from build123d import *

# Parameters (mm, degrees)
SKETCH1_W           = 26
SKETCH1_H           = 26
SKETCH1_R           = 1.5
BOSS_EXTRUDE1_DEPTH = 20
SKETCH2_R           = 10
SKETCH2_R_2         = 3
CUT_EXTRUDE1_DEPTH  = 15
SKETCH2_7_R         = 3
SKETCH2_7_R_2       = 1.5
CUT_EXTRUDE3_DEPTH  = 17
CHAMFER1_SIZE       = 1
BOSS_EXTRUDE3_DEPTH = 3.5


with BuildPart() as part:
    # Sketch1 → Boss-Extrude1 (new body)
    with BuildSketch(Plane.XY):
        with Locations((2.653979239, -3.148788927)):
            Rectangle(SKETCH1_W, SKETCH1_H)
        with Locations((2.653979239, 2.851211073)):
            Circle(SKETCH1_R, mode=Mode.SUBTRACT)
        with Locations((2.653979239, -9.148788927)):
            Circle(SKETCH1_R, mode=Mode.SUBTRACT)
    extrude(amount=BOSS_EXTRUDE1_DEPTH)

    # Sketch2 → Cut-Extrude1 (cut)
    with BuildSketch(Plane(origin=(0, 0, 0), x_dir=(-1, 0, 0), z_dir=(0, 0, -1))):
        with Locations((-2.653979239, -3.148788927)):
            Circle(SKETCH2_R)
        with Locations((-2.653979239, 2.851211073)):
            Circle(SKETCH2_R_2, mode=Mode.SUBTRACT)
        with Locations((-2.653979239, -9.148788927)):
            Circle(SKETCH2_R_2, mode=Mode.SUBTRACT)
    extrude(amount=-CUT_EXTRUDE1_DEPTH, mode=Mode.SUBTRACT)

    # Sketch2_7 → Cut-Extrude3 (cut)
    # profile 1 of 2: a face of its own
    with BuildSketch(Plane(origin=(0, 0, 0), x_dir=(-1, 0, 0), z_dir=(0, 0, -1))):
        with Locations((-2.653979239, 2.851211073)):
            Circle(SKETCH2_7_R)
        with Locations((-2.653979239, 2.851211073)):
            Circle(SKETCH2_7_R_2, mode=Mode.SUBTRACT)
    # profile 2 of 2: a face of its own
    with BuildSketch(Plane(origin=(0, 0, 0), x_dir=(-1, 0, 0), z_dir=(0, 0, -1))):
        with Locations((-2.653979239, -9.148788927)):
            Circle(SKETCH2_7_R)
        with Locations((-2.653979239, -9.148788927)):
            Circle(SKETCH2_7_R_2, mode=Mode.SUBTRACT)
    extrude(amount=-CUT_EXTRUDE3_DEPTH, mode=Mode.SUBTRACT)

    # Chamfer1
    chamfer1_edges = [part.edges().sort_by_distance(p)[0] for p in [
        (2.653979239, 9.851211073, 0),
        (15.653979239, -3.148788927, 0),
        (2.653979239, -16.148788927, 0),
        (-10.346020761, -3.148788927, 0),
    ]]
    chamfer(chamfer1_edges, length=CHAMFER1_SIZE)

    # Sketch3 → Boss-Extrude3 (add)
    with BuildSketch(Plane(origin=(0, 0, 0), x_dir=(-1, 0, 0), z_dir=(0, 0, -1))):
        with BuildLine():
            Line((5.043710991, 3.466589231), (1.49333202, 0))
            ThreePointArc((1.49333202, 0), (2.221785028, -1.395131682), (2.473152007, -2.948788927))
            ThreePointArc((2.473152007, -2.948788927), (2.221785028, -4.502446173), (1.49333202, -5.897577855))
            Line((1.49333202, -5.897577855), (5.043710991, -9.364167085))
            Line((5.043710991, -9.364167085), (5.524107903, -9.77521739))
            ThreePointArc((5.524107903, -9.77521739), (8.045991974, -2.924201539), (5.492050202, 3.914928442))
            Line((5.492050202, 3.914928442), (5.043710991, 3.466589231))
        make_face()
        with BuildLine():
            ThreePointArc((-6.401290497, -5.897577855), (-7.381110484, -2.948788927), (-6.401290497, 0))
            Line((-6.401290497, 0), (-9.951669468, 3.466589231))
            Line((-9.951669468, 3.466589231), (-10.43206638, 3.877639536))
            ThreePointArc((-10.43206638, 3.877639536), (-12.953812767, -2.889662973), (-10.508439041, -9.684935993))
            Line((-10.508439041, -9.684935993), (-10.124893336, -9.364167085))
            Line((-10.124893336, -9.364167085), (-6.401290497, -5.897577855))
        make_face()
    extrude(amount=-BOSS_EXTRUDE3_DEPTH)


solid = part.part
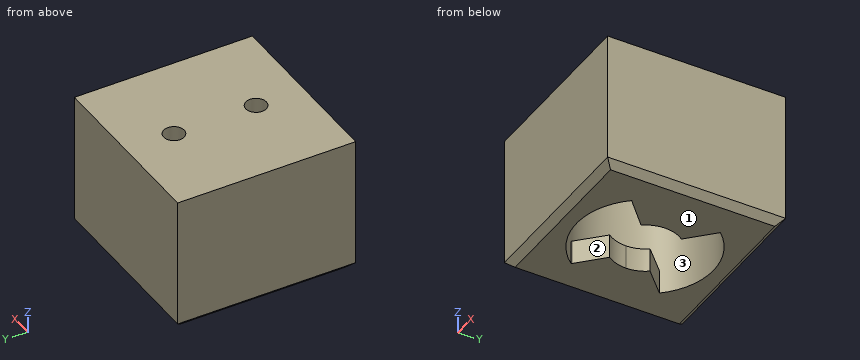
Here's how the part is built. I have some questions about the finished solid (model axes, mm). Face numbers are marked on the shaded views. Round coordinates to 2 decimals unless told otherwise and drop trailing zeros. Write each loop counter-clockwise with the first axis right and the second up, starting at its lowest first coordinate (ties: lowest second). Pieces come first, ordered by that corner, then holes.
1. Suppose I cut it at B-B (x = -6). List the corners of the cut face in (y, z) for me, and give its area (3 significant figures).
2. If we mould it in two halves opening along Z, with no side actions, what happens to the marked faces 1, 2 and 3? For each: released by +Z, released by -Z, zero draft, split by the parting line, or undercut.
3. Suppose I cut it at A-A (x = 2.25). List the corners of the cut face in (y, z) for me.
4. I need wall thicknesses on L1, parallel to Z at x = -7, y = -1; L2, parallel to X at y = -3.5, z = 13.75; L3, parallel to Y at x = 3, z = 7. Which ranges of each line are inside material? Lowest first, please.
5. Will these pins go through, and if not, where does the flat tip stop? pin 1 Ø5 at (x, y) = (2, -10) entering from -Z; pin 2 Ø5.5 at (x, y) = (2.65, -9.15) entering from -Z.
6. Suppose I cut it at D-D (y = -7.25). List the corners of the cut face in (x, z) for me.
7. Suppose I cut it at C-C (z = 13.75). List the corners of the cut face in (x, y) for me, and give its area (3 significant figures).
Answer sheet:
1. outline: (-16.15, 1) - (-15.15, 0) - (8.85, 0) - (9.85, 1) - (9.85, 20) - (-16.15, 20) - close; hole (-8.16, 3.5) - (1.86, 3.5) - (1.86, 15) - (-8.16, 15) - close
1. area: 404 mm2
2. face 1: released by -Z
2. face 2: zero draft
2. face 3: undercut
3. outline: (-16.15, 1) - (-15.15, 0) - (-13.14, 0) - (-13.14, 15) - (-12.12, 15) - (-12.12, 17) - (-10.59, 17) - (-10.59, 20) - (-16.15, 20) - close; (-7.7, 17) - (-6.18, 17) - (-6.18, 15) - (-0.12, 15) - (-0.12, 17) - (1.41, 17) - (1.41, 20) - (-7.7, 20) - close; (4.3, 17) - (5.82, 17) - (5.82, 15) - (6.84, 15) - (6.84, 0) - (8.85, 0) - (9.85, 1) - (9.85, 20) - (4.3, 20) - close
4. L1: z = 0 to 3.5, 15 to 20
4. L2: x = -10.35 to -7.34, 12.65 to 15.65
4. L3: y = -16.15 to -13.14, 6.85 to 9.85
5. pin 1: stops at z = 15
5. pin 2: stops at z = 17
6. outline: (-10.35, 1) - (-9.35, 0) - (-2.88, 0) - (-2.88, 3.5) - (-6.47, 3.5) - (-6.47, 15) - (0.33, 15) - (0.33, 17) - (4.98, 17) - (4.98, 15) - (11.77, 15) - (11.77, 3.5) - (7.85, 3.5) - (7.85, 0) - (14.65, 0) - (15.65, 1) - (15.65, 20) - (-10.35, 20) - close
7. outline: (-10.35, -16.15) - (15.65, -16.15) - (15.65, 9.85) - (-10.35, 9.85) - close; hole circle Ø20 at (2.65, -3.15)
7. area: 362 mm2
